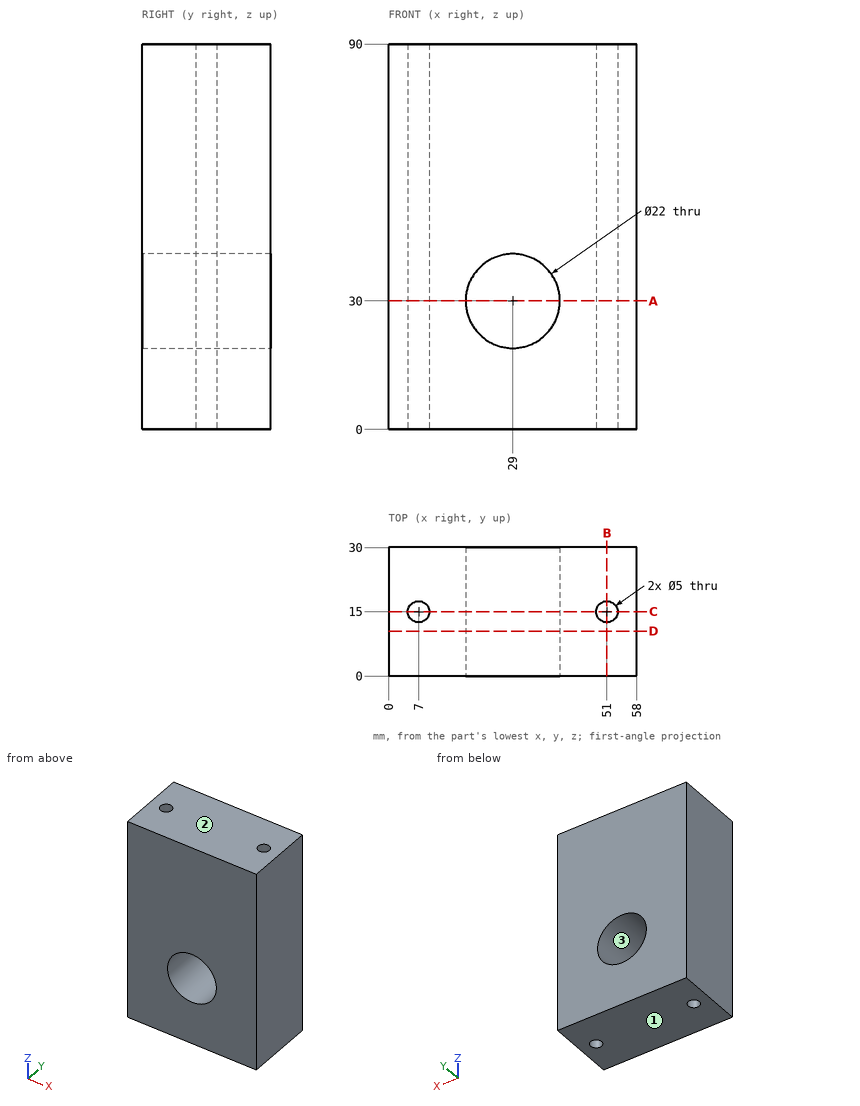
For this review, use the dimensioned drawing (mm, ordinates from the lowest corner) and the shaded views. Coordinates: 2 decimals unless noted, no trailing zeros. Write each loop counter-clockwise with the first axis right and the second up, starting at its lowest first coordinate (ties: lowest second). Pieces come first, ordered by that corner, then holes. Notation, with made-up numbers: (52.5, -14) - (59.5, -14) arc R28 cw to (59.5, 18) - close; hole circle Ø9 at (33.25, 5). An arc over 180 degrees is marked (long way). Answer as a JSON object with one key per item and string values. Group by question number.
1. Add section B-B (x = 51). Give the boundary of the cut face in (y, z), plus the area to 3 significant figures.
2. Add section D-D (y = 10.5). Give the boundary of the cut face in (x, z), plus the area to 3 significant figures.
3. Mouldability with a two-part tool opening along Z and no side actions: class the marked faces 1, 2 and 3 as pulls with the +Z half, pulls with the -Z half, needs draft (parallel to the pull), parting line crosses it, or undercut.
4. To check wall thickness, follow probe 1 along Y at (x, z) = (51, 46); probe 2 along X at (y, z) = (13.5, 43); probe 3 along Z at (x, y) = (26, 23). State the ranges of each line that lie inside material, in increasing order.
5. Add section C-C (y = 15). Give the boundary of the cut face in (x, z), plus the area to 3 significant figures.
6. Add section A-A (z = 30). Give the boundary of the cut face in (x, y).
Findings:
{
 "1": {"outline": "(0, 0) - (12.5, 0) - (12.5, 90) - (0, 90) - close; (17.5, 0) - (30, 0) - (30, 90) - (17.5, 90) - close", "area": "2,250 mm²"},
 "2": {"outline": "(0, 0) - (58, 0) - (58, 90) - (0, 90) - close; hole circle Ø22 at (29, 30)", "area": "4,840 mm²"},
 "3": {"face 1": "pulls with the -Z half", "face 2": "pulls with the +Z half", "face 3": "undercut"},
 "4": {"probe 1": "0 to 12.5, 17.5 to 30", "probe 2": "0 to 5, 9 to 49, 53 to 58", "probe 3": "0 to 19.42, 40.58 to 90"},
 "5": {"outline": "(0, 0) - (4.5, 0) - (4.5, 90) - (0, 90) - close; (9.5, 0) - (48.5, 0) - (48.5, 90) - (9.5, 90) - close; (53.5, 0) - (58, 0) - (58, 90) - (53.5, 90) - close; hole circle Ø22 at (29, 30)", "area": "3,940 mm²"},
 "6": {"outline": "(0, 0) - (18, 0) - (18, 30) - (0, 30) - close; (40, 0) - (58, 0) - (58, 30) - (40, 30) - close; hole circle Ø5 at (7, 15); hole circle Ø5 at (51, 15)"}
}
